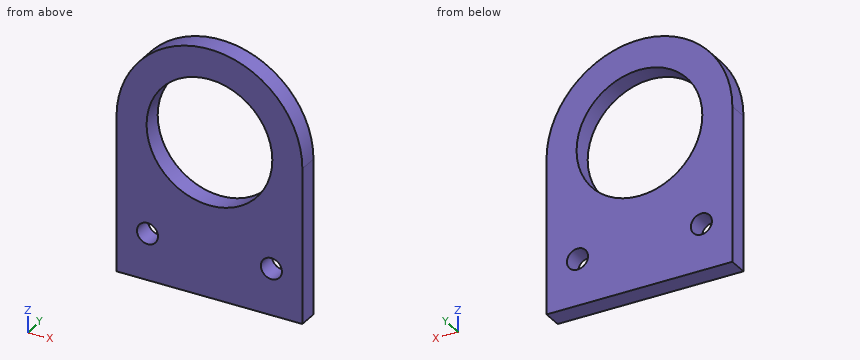
```python
from build123d import *

# Parameters (mm, degrees)
F0_R     = 4.318
F0_R_2   = 25.781
F1_DEPTH = 7.9375


with BuildPart() as f1:
    # F0 (on Front) → F1 (new body)
    with BuildSketch(Plane.XZ):
        with BuildLine():
            Line((38.1, -63.5), (38.1, 0))
            ThreePointArc((38.1, 0), (0, 38.1), (-38.1, 0))
            Line((-38.1, 0), (-38.1, -63.5))
            Line((-38.1, -63.5), (38.1, -63.5))
        make_face()
        with Locations((-25.4, -44.45)):
            Circle(F0_R, mode=Mode.SUBTRACT)
        with Locations((25.4, -44.45)):
            Circle(F0_R, mode=Mode.SUBTRACT)
        Circle(F0_R_2, mode=Mode.SUBTRACT)
    extrude(amount=F1_DEPTH)


solid = f1.part
```
Read the model definition and answer for the solid it produces. Units are mm, in the model's axes. Give positions to 0.01 mm unless a question says otherwise; leave off trailing zeros. Write each loop counter-clockwise with the first axis right and the second up, starting at its lowest first coordinate (ties: lowest second). Pieces come first, ordered by that corner, then holes. Notation, with made-up numbers: (69, 54.25) - (74, 54.25) arc R5 cw to (74, 58.25) - close; hole circle Ø5 at (37, -13.5). An arc over 180 degrees is marked (long way). Write item = value, one per line. Start each with the question number.
Item 1: Find section A-A (z = -44.45). Give the vertices of the cut face in (x, y).
Item 2: Find the intervals of material crossed by probe 1 along Z at (x, y) = (0, -3.75); probe 2 along Z at (x, y) = (23, -6.75); probe 3 along X at (y, z) = (-0.5, -48), in increasing order. Write a range as [from, to].
Item 3: Find section D-D (z = -21). Give the vertices of the cut face in (x, y).
Item 4: Find section C-C (y = -6.5). Give the vertices of the cut face in (x, z).
Item 5: Each of these flat-tipped pins is pushed along its axis until it touches: P1, Ø14, axis at x = -25.4, z = -44.45, coming from the +Y side; P2, Ø3, axis at x = 10.5, y = -4.5, coming from the +Z side; P3, Ø3, axis at y = -6, z = 14, coming from the -X side; P4, Ø6, axis at x = -21.5, z = 4.5, coming from the +Y side. Where does it stop, or does it pass through?
Item 6: Find section B-B (x = 18). Give the vertices of the cut face in (y, z), then the cut area to 3 significant figures.
Response:
q1.outline = (-38.1, -7.94) - (-29.72, -7.94) - (-29.72, 0) - (-38.1, 0) - close; (-21.08, -7.94) - (21.08, -7.94) - (21.08, 0) - (-21.08, 0) - close; (29.72, -7.94) - (38.1, -7.94) - (38.1, 0) - (29.72, 0) - close
q2.probe_1 = [-63.5, -25.78], [25.78, 38.1]
q2.probe_2 = [-63.5, -48.04], [-40.86, -11.65], [11.65, 30.37]
q2.probe_3 = [-38.1, -27.86], [-22.94, 22.94], [27.86, 38.1]
q3.outline = (-38.1, -7.94) - (-14.96, -7.94) - (-14.96, 0) - (-38.1, 0) - close; (14.96, -7.94) - (38.1, -7.94) - (38.1, 0) - (14.96, 0) - close
q4.outline = (-38.1, -63.5) - (38.1, -63.5) - (38.1, 0) arc R38.1 ccw to (-38.1, 0) - close; hole circle Ø8.64 at (-25.4, -44.45); hole circle Ø51.56 at (0, 0); hole circle Ø8.64 at (25.4, -44.45)
q5.P1 = 0
q5.P2 = 37.02
q5.P3 = -35.99
q5.P4 = through
q6.outline = (-7.94, -63.5) - (0, -63.5) - (0, -18.46) - (-7.94, -18.46) - close; (-7.94, 18.46) - (0, 18.46) - (0, 33.58) - (-7.94, 33.58) - close
q6.area = 478 mm²
